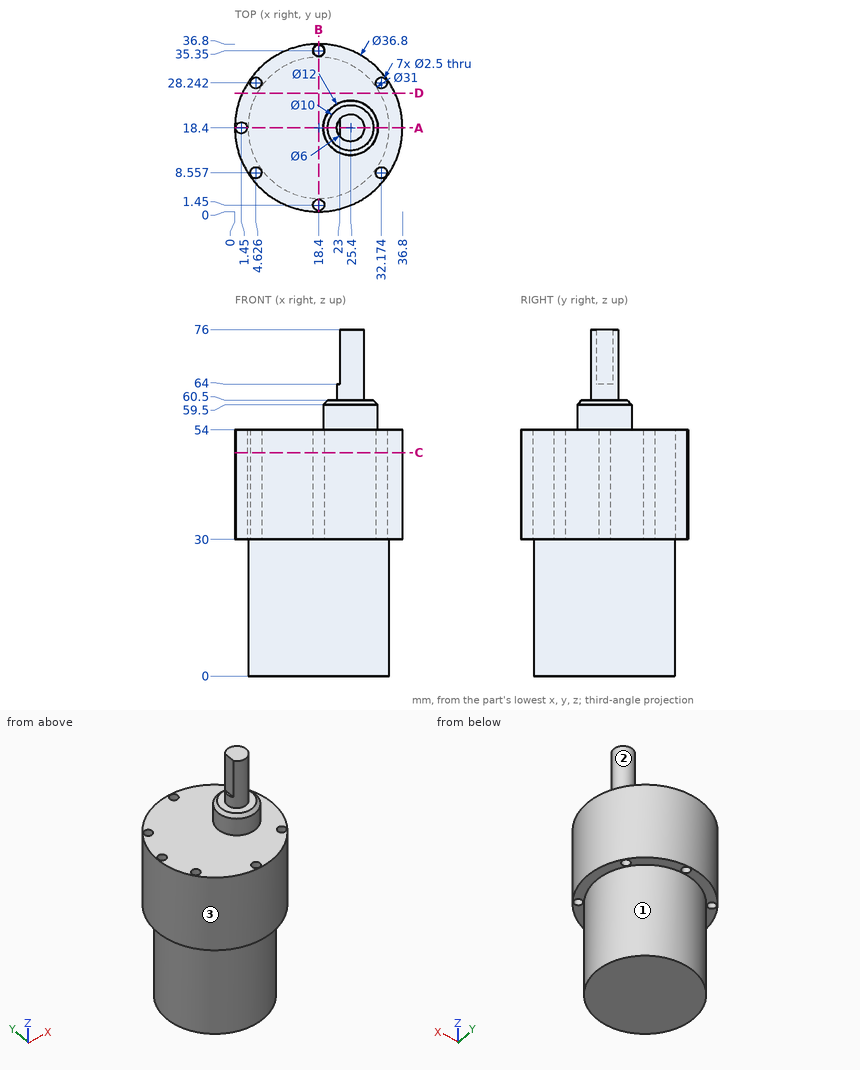
Answer from the drawing. Dimensions are ordinates in mm from the lowest x, y and z of the part. A direction names the side the tool comes from. Round coordinates to 2 decimals unless told otherwise and drop trailing zeros. Loops run counter-clockwise (first coordinate to the right, second up) from the corner with the lowest first, then second, coordinate; pieces in that order, holes last.
Q1. Section A-A on y = 18.4 is taken. Write down the section's boundary in (x, z).
Q2. Section B-B on x = 18.4 is taken. Write down the section's boundary in (y, z).
Q3. Consider probe 1 along Y at (x, z) = (18.4, 39.5); probe 2 along Y at (x, z) = (18, 39) (1 decimal); probe 3 along Z at (x, y) = (10, 14). Determine where each line is inside the solid, lowest interval first.
Q4. Which of the six approach directions +Z, -Z, +X, -X, +Y, -Y give full straight-line access (tool end or side, diameter ignored) to the marked faces 1, 2 and 3?
Q5. Section D-D on y = 26 is taken. Write down the section's boundary in (x, z).
Q6. Each of these flat-tipped pins is pushed along its axis until it touches: pin 1 (3 mm diameter, centred on x = 32.17, y = 8.56, fed in from -Z); pin 2 (11 mm diameter, centred on x = 11.5, y = 18, fed in from +Z); pin 3 (1.5 mm diameter, centred on y = 32.5, z = 11, fed in from -X) (1 decimal); pin 4 (1 mm diameter, centred on y = 13.5, z = 14.5, fed in from -X). Where does it stop, or does it pass through?
Q7. Section C-C on z = 49 is taken. Give the number of separate pieces and of enclosed holes in the cut face, and give its area (3 significant figures).
Output:
1. outline: (0, 30) - (0.2, 30) - (0.2, 54) - (0, 54) - close; (2.7, 30) - (2.9, 30) - (2.9, 0) - (33.9, 0) - (33.9, 30) - (36.8, 30) - (36.8, 54) - (31.4, 54) - (31.4, 59.5) - (30.4, 60.5) - (28.4, 60.5) - (28.4, 76) - (23, 76) - (23, 64) - (22.4, 64) - (22.4, 60.5) - (20.4, 60.5) - (19.4, 59.5) - (19.4, 54) - (2.7, 54) - close
2. outline: (0, 30) - (0.2, 30) - (0.2, 54) - (0, 54) - close; (2.7, 30) - (2.9, 30) - (2.9, 0) - (33.9, 0) - (33.9, 30) - (34.1, 30) - (34.1, 54) - (2.7, 54) - close; (36.6, 30) - (36.8, 30) - (36.8, 54) - (36.6, 54) - close
3. probe 1: y = 0 to 0.2, 2.7 to 34.1, 36.6 to 36.8
3. probe 2: y = 0 to 0.3, 2.6 to 34.2, 36.5 to 36.8
3. probe 3: z = 0 to 54
4. face 1: -Z
4. face 2: +Z
4. face 3: +Z, -Z
5. outline: (1.64, 30) - (4.89, 30) - (4.89, 0) - (31.91, 0) - (31.91, 30) - (35.16, 30) - (35.16, 54) - (1.64, 54) - close
6. pin 1: stops at z = 0
6. pin 2: stops at z = 54
6. pin 3: stops at x = 10.5
6. pin 4: stops at x = 3.54
7. separate pieces: 1
7. enclosed holes: 7
7. area: 1,030 mm2
